Build history of the part. All positions in model axes, mm. Give positions to 0.01 mm unless a question says otherwise; leave off trailing zeros. Order: outer loops, then holes, each group sorted by start corner. A loop starts at its lowest first (then second) coordinate and runs counter-clockwise, first axis right, second up. Notation, with made-up numbers: M 41.5,-20.5 L 71.5,-20.5 A10 ccw 71.5,-11.5 Z; hole C 3,23 d7. An arc over 180 degrees is marked long. Use CSV: the item, a comma, the result in double quotes. Start each with the question number.
Item 1: Band-saw the part on B-B on y = 278. Write the cut outline in (x, z) (1 decimal).
Item 2: Band-saw the part on C-C on x = 1672. Write the cut outline in (y, z) (1 decimal).
Item 3: Band-saw the part on D-D on x = 0. Give the number of separate pieces and of enclosed holes in the cut face, plus the area to 3 significant figures.
Item 4: Wall check: line 1 along Z through (x, y) = (0, 268.5); line 2 along Y through (x, z) = (403, 1). Give the ranges that are in metal, low to high.
Item 5: Band-saw the part on A-A on z = 0. Write the cut outline in (x, y) (1 decimal).
Item 6: Two-plate mould, pull along X, no slides. Class faces 1 (the cylindrical face through (-60.47, 197.877, 46.367)), 2 (the cylindrical face through (1155.446, 529.348, -25.273)), 3 (the cylindrical face through (-18.239, 180.289, 82.137)): pulls with the +X half, pulls with the -X half, needs draft (parallel to the pull), parting line crosses it, or undercut.
Item 7: Pin check, flat tips, straight feed: P1, Ø2, axis at x = 408, z = 6.5, coming from the +Y side; P2, Ø3, axis at x = 1203.5, z = -49, coming from the +Y side; P3, Ø4, axis at x = 543, z = 48.5, coming from the +Y side. Stop position of each tip, or through.
from build123d import *

# Parameters (mm, degrees)
F1_R   = 84.1375
F1_R_2 = 76.2


with BuildPart() as f2:
    # F2: sweep along a path in F0
    with BuildLine(Plane.XY) as f2_path:
        Line((0, 0), (0, 355.6))
        ThreePointArc((0, 355.6), (74.3948775786, 535.2051224214), (254, 609.6))
        Line((254, 609.6), (2032, 609.6))
    # F1 (on Front) → F2 (sweep)
    with BuildSketch(Plane.XZ):
        Circle(F1_R)
        Circle(F1_R_2, mode=Mode.SUBTRACT)
    sweep(path=f2_path.line)

    # F3 (on Top) → F4 (revolve)
    with BuildSketch(Plane.XY):
        with BuildLine():
            Line((-76.2, 0), (-84.1375, 0))
            ThreePointArc((-84.1375, 0), (0, -84.1375), (84.1375, 0))
            Line((84.1375, 0), (76.2, 0))
            ThreePointArc((76.2, 0), (0, -76.2), (-76.2, 0))
        make_face()
    revolve(axis=Axis((0, 0, 0), (1, 0, 0)))

    # F5 (on face) → F6 (revolve)
    with BuildSketch(Plane.YZ.offset(2032)):
        with BuildLine():
            Line((533.4, 0), (609.6, 0))
            Line((609.6, 0), (685.8, 0))
            ThreePointArc((685.8, 0), (609.6, 76.2), (533.4, 0))
        make_face()
        with BuildLine():
            Line((525.4625, 0), (533.4, 0))
            ThreePointArc((533.4, 0), (609.6, 76.2), (685.8, 0))
            Line((685.8, 0), (693.7375, 0))
            ThreePointArc((693.7375, 0), (609.6, 84.1375), (525.4625, 0))
        make_face()
    revolve(axis=Axis((2032, 625.8413642645, 0), (0, 1, 0)))


solid = f2.part
Model answer:
1,outline,"C 0,0 d168.3; hole C 0,0 d152.4"
2,outline,"C 609.6,0 d168.3; hole C 609.6,0 d152.4"
3,separate pieces,"1"
3,enclosed holes,"2"
3,area,"13,900 mm^2"
4,line 1,"z = -84.14 to -76.2, 76.2 to 84.14"
4,line 2,"y = 525.47 to 533.41, 685.79 to 693.73"
5,outline,"M -84.1,0 A84.1 ccw 84.1,0 L 84.1,355.6 A169.9 cw 254,525.5 L 2032,525.5 A84.1 ccw 2032,693.7 L 254,693.7 A338.1 ccw -84.1,355.6 Z; hole C 0,0 d152.4; hole M -76.2,35.7 A84.1 cw 76.2,35.7 L 76.2,355.6 A177.8 cw 254,533.4 L 1996.3,533.4 A84.1 cw 1996.3,685.8 L 254,685.8 A330.2 ccw -76.2,355.6 Z"
6,face 1,"undercut"
6,face 2,"needs draft"
6,face 3,"parting line crosses it"
7,P1,"stops at y = 693.56"
7,P2,"stops at y = 679.05"
7,P3,"stops at y = 679.72"
